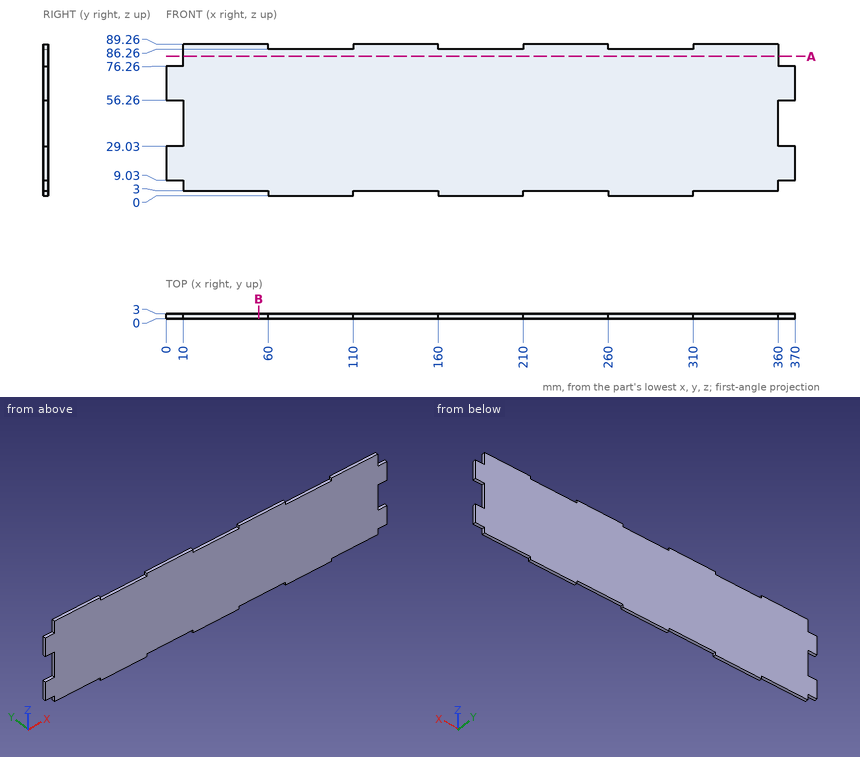
The drawing under review shows one solid part. Ordinate dimensions are in mm from its lowest x, y, z. Give positions to 0.01 mm unless a question says otherwise; leave off trailing zeros. Loops run counter-clockwise (first coordinate to the right, second up) from the corner with the lowest first, then second, coordinate; pieces in that order, holes last. Notation, with made-up numbers: M -8,-25 L 5,-25 A24 ccw 5,-8 Z; hole C 82.25,1 d7. An arc over 180 degrees is marked long. Return JSON: item names as keys, results as strings. Group by question number.
Item 1: Insertion check: pin 1 Ø0.9 at (x, y) = (293, 2) entering from +Z; pin 2 Ø0.9 at (y, z) = (1.5, 1) entering from +X; pin 3 Ø1.5 at (y, z) = (2, 88) entering from -X. Each pin has a flat end and moves straight along its axis. Give the tip position at first contact, or say it passes through.
Item 2: For probe 1 along Z at (x, y) = (34, 2.55); probe 2 along Z at (x, y) = (96, 1.3); probe 3 along X at (y, z) = (2.8, 38.5), list the stretches that pass through material, from the lowest coordinate up.
Item 3: We need section B-B (x = 54.5). Give the boundary of the cut face in (y, z), and give its area (3 significant figures).
Item 4: We need section A-A (z = 82). Give the boundary of the cut face in (x, y).
Output:
{
 "1": {"pin 1": "stops at z = 86.26", "pin 2": "stops at x = 310", "pin 3": "stops at x = 10"},
 "2": {"probe 1": "z = 3 to 89.26", "probe 2": "z = 0 to 86.26", "probe 3": "x = 10 to 360"},
 "3": {"outline": "M 0,3 L 3,3 L 3,89.26 L 0,89.26 Z", "area": "259 mm^2"},
 "4": {"outline": "M 10,0 L 360,0 L 360,3 L 10,3 Z"}
}
